from build123d import *

# Parameters (mm, degrees)
ESBO_O1_R                       = 5.82
RESSALTO_EXTRUS_O1_DEPTH        = 60.8
ESBO_O2_R                       = 11
RESSALTO_EXTRUS_O2_DEPTH        = 12
FILETE1_R                       = 2
CORTE_EXTRUS_O1_DEPTH           = 10.4
ESBO_O4_R                       = 3.7
CORTE_EXTRUS_O2_DEPTH           = 61
ESBO_O5_R                       = 2
CORTE_EXTRUS_O3_DEPTH           = 2
FILETE2_R                       = 2
VARREDURA_DE_CORTE1_PITCH       = 2
VARREDURA_DE_CORTE1_HEIGHT      = 10.4
VARREDURA_DE_CORTE1_RADIUS      = 5.82
VARREDURA_DE_CORTE1_START_ANGLE = -180
ESBO_O10_OUTSIDE_W              = 39.834
ESBO_O10_OUTSIDE_H              = 39.834
ESBO_O10_OUTSIDE_R              = 8.2
CORTE_EXTRUS_O4_DEPTH           = 10.4
FILETE3_R                       = 1
CORTE_EXTRUS_O6_DEPTH           = 10


with BuildPart() as part:
    # Esboço1 → Ressalto-extrusão1 (new body)
    with BuildSketch(Plane(origin=(0, 0, 0), x_dir=(1, 0, 0), z_dir=(0, 1, 0))):
        Circle(ESBO_O1_R)
    extrude(amount=RESSALTO_EXTRUS_O1_DEPTH)

    # Esboço2 → Ressalto-extrusão2 (add)
    with BuildSketch(Plane(origin=(0, 60.8, 0), x_dir=(1, 0, 0), z_dir=(0, 1, 0))):
        Circle(ESBO_O2_R)
    extrude(amount=RESSALTO_EXTRUS_O2_DEPTH)

    # Filete1
    filete1_edges = [part.edges().sort_by_distance(p)[0] for p in [
        (-5.82, 60.8, 0),
    ]]
    fillet(filete1_edges, radius=FILETE1_R)

    # Esboço3 → Corte-extrusão1 (cut)
    with BuildSketch(Plane(origin=(0, 72.8, 0), x_dir=(1, 0, 0), z_dir=(0, 1, 0))):
        Polygon((-7.390083446, 0), (-3.695041723, -6.4), (3.695041723, -6.4), (7.390083446, 0), (3.695041723, 6.4), (-3.695041723, 6.4), align=None)
    extrude(amount=-CORTE_EXTRUS_O1_DEPTH, mode=Mode.SUBTRACT)

    # Esboço4 → Corte-extrusão2 (cut)
    with BuildSketch(Plane.XZ):
        Circle(ESBO_O4_R)
    extrude(amount=-CORTE_EXTRUS_O2_DEPTH, mode=Mode.SUBTRACT)

    # Esboço5 → Corte-extrusão3 (cut)
    with BuildSketch(Plane(origin=(0, 62.4, 0), x_dir=(1, 0, 0), z_dir=(0, 1, 0))):
        Circle(ESBO_O5_R)
    extrude(amount=-CORTE_EXTRUS_O3_DEPTH, mode=Mode.SUBTRACT)

    # Filete2
    filete2_edges = [part.edges().sort_by_distance(p)[0] for p in [
        (-5.82, 0, 0),
    ]]
    fillet(filete2_edges, radius=FILETE2_R)

    # Varredura de corte1: sweep along a helix
    with BuildLine() as varredura_de_corte1_path:
        add(Helix(VARREDURA_DE_CORTE1_PITCH, VARREDURA_DE_CORTE1_HEIGHT, VARREDURA_DE_CORTE1_RADIUS, center=(0, 0, 0), direction=(0, 1, 0), mode=Mode.PRIVATE).rotate(Axis((0, 0, 0), (0, 1, 0)), VARREDURA_DE_CORTE1_START_ANGLE))
    # Esboço9 → Varredura de corte1 (sweep, cut)
    with BuildSketch(Plane(origin=(0, 0, 0), x_dir=(0, 0, -1), z_dir=(1, 0, 0))):
        Polygon((4.5198, 0), (6.4698, -1.125833025), (6.4698, 1.125833025), align=None)
    sweep(path=varredura_de_corte1_path.line, is_frenet=True, mode=Mode.SUBTRACT)

    # Esboço10 outside → Corte-extrusão4 (cut)
    with BuildSketch(Plane(origin=(0, 72.8, 0), x_dir=(1, 0, 0), z_dir=(0, 1, 0))):
        Rectangle(ESBO_O10_OUTSIDE_W, ESBO_O10_OUTSIDE_H)
        Circle(ESBO_O10_OUTSIDE_R, mode=Mode.SUBTRACT)
    extrude(amount=-CORTE_EXTRUS_O4_DEPTH, mode=Mode.SUBTRACT)

    # Filete3
    filete3_edges = [part.edges().sort_by_distance(p)[0] for p in [
        (-8.2, 62.4, 0),
    ]]
    fillet(filete3_edges, radius=FILETE3_R)

    # Esboço12 → Corte-extrusão6 (cut)
    with BuildSketch(Plane(origin=(0, 0, 0), x_dir=(-0.951056516, 0, -0.309016994), z_dir=(0.309016994, 0, -0.951056516))):
        Polygon((5.82, 9.64932918), (5.82, 11.15067082), (4.5198, 10.4), align=None)
    extrude(amount=-CORTE_EXTRUS_O6_DEPTH, mode=Mode.SUBTRACT)


solid = part.part
Design review of the part built by this model. Coordinates are the model's own, in mm. A direction names the side the tool comes from. Round coordinates to 2 decimals unless told otherwise and drop trailing zeros. Loops run counter-clockwise (first coordinate to the right, second up) from the corner with the lowest first, then second, coordinate; pieces in that order, holes last. Notation, with made-up numbers: M 9.5,-7 L 16.5,-7 A20 ccw 16.5,15 Z; hole C -4,-0.5 d6. An arc over 180 degrees is marked long. Answer as a JSON object with one key per item and string values.
Item 1: Clearance check with flat-ended pins moving along their axes: P1, Ø6.5, axis at x = 0, z = -0.5, coming from the -Y side; P2, Ø1.5, axis at x = 5, z = 7, coming from the -Y side; P3, Ø5, axis at x = -7.5, y = 21, coming from the +Z side; P4, Ø4, axis at y = 60, z = -5.5, coming from the +X side. State where each tip first meets the part, or that it passes through.
Answer sheet:
{"P1": "stops at y = 0", "P2": "stops at y = 60.8", "P3": "stops at z = 2.98", "P4": "stops at x = 10.37"}
Item 2: The part is to be moulded in two halves that separate along X. For faces 4 (the flat face through (0, 68, -6.4)), 5 (the cylindrical face through (-2.38, 61.59, 10.74)), 6 (the flat face through (5, 62.4, 8)), say which applies: pulls with the +X half, pulls with the -X half, needs draft (parallel to the pull), parting line crosses it, or undercut.
Answer sheet:
{"face 4": "undercut", "face 5": "parting line crosses it", "face 6": "needs draft"}
Item 3: We need section A-A on y = 49. Give the boundary of the cut face in (x, z), and give its area (3 significant figures).
Answer sheet:
{"outline": "C 0,0 d11.64; hole C 0,0 d7.4", "area": "63.4 mm^2"}
Item 4: Wall thickness on L1, parallel to Z at x = 0, y = 61.4; L2, parallel to Y at x = -1.5, z = 4.5: over which ranges is each line inside the solid? List them lowest first. Write a range as from..to.
Answer sheet:
{"L1": "z = -11..-2, 2..11", "L2": "y = 0.23..0.77, 1.03..2.77, 3.03..4.77, 5.03..6.77, 7.03..8.77, 9.03..62.4"}
Item 5: Machinability: for faces 1 (the flat face through (-5.568, 67.673, 3.155)), 2 (the flat face through (-6, 72.8, -4)), 3 (the flat face through (7, 60.8, 5)), which of the approach directions +Z, -Z, +X, -X, +Y, -Y give a long, thin tool a straight path to every point of the face, cutting with its end or side? Answer none if there is none.
Answer sheet:
{"face 1": "+Y", "face 2": "+Z, -Z, +X, -X, +Y", "face 3": "-Y"}
